from build123d import *

# Parameters (mm, degrees)
SKETCH_W     = 380
SKETCH_H     = 250
PAD_DEPTH    = 18
SKETCH001_W  = 284
SKETCH001_H  = 154
POCKET_DEPTH = 5
SKETCH004_R  = 1.55
HOLE_DEPTH   = 13.001


with BuildPart() as part:
    # Sketch → Pad (new body)
    with BuildSketch(Plane.XY):
        with Locations((190, 125)):
            Rectangle(SKETCH_W, SKETCH_H)
    extrude(amount=PAD_DEPTH)

    # Sketch001 (on Face6 of Pad) → Pocket (cut)
    with BuildSketch(Plane.XY.offset(18)):
        Polygon((30, 250), (30, 220), (0, 220), (0, 202), (30, 202), (30, 48), (0, 48), (0, 30), (30, 30), (30, 0), (48, 0), (48, 30), (332, 30), (332, 0), (350, 0), (350, 30), (380, 30), (380, 48), (350, 48), (350, 202), (380, 202), (380, 220), (350, 220), (350, 250), (332, 250), (332, 220), (48, 220), (48, 250), align=None)
        with Locations((190, 125)):
            Rectangle(SKETCH001_W, SKETCH001_H, mode=Mode.SUBTRACT)
    extrude(amount=-POCKET_DEPTH, mode=Mode.SUBTRACT)

    # Sketch004 (on Face6 of Pocket) → Hole (cut, through all)
    with BuildSketch(Plane.XY.offset(13)):
        with Locations((39, 39)):
            Circle(SKETCH004_R)
        with Locations((341, 39)):
            Circle(SKETCH004_R)
        with Locations((341, 211)):
            Circle(SKETCH004_R)
        with Locations((39, 211)):
            Circle(SKETCH004_R)
        with Locations((190, 211)):
            Circle(SKETCH004_R)
        with Locations((190, 39)):
            Circle(SKETCH004_R)
    extrude(amount=-HOLE_DEPTH, mode=Mode.SUBTRACT)


solid = part.part
Can you work these out from the model? Positions are in its coordinate system, mm. Give positions to 0.01 mm unless a question says otherwise; leave off trailing zeros. Order: outer loops, then holes, each group sorted by start corner. A loop starts at its lowest first (then second) coordinate and runs counter-clockwise, first axis right, second up. Notation, with made-up numbers: (-28, 74.5) - (-3, 74.5) arc R22 ccw to (-3, 89.5) - close; hole circle Ø8 at (81, 64). An arc over 180 degrees is marked (long way). Write each question's results on one line, items separated by ' | '.
1) I'm going to push a flat-ended pin straight in: pin 1 Ø4 at (x, z) = (361, 16) entering from -Y. Where does the tip first touch, or does it pass through?
Final values:
pin 1: stops at y = 0
2) Please list where these lines run through material, in increasing order: line 1 along X through (y, z) = (211, 9.5); line 2 along X through (y, z) = (12.5, 15); line 3 along Y through (x, z) = (190, 3.75). Write a range as [from, to].
Final values:
line 1: x = [0, 37.45], [40.55, 188.45], [191.55, 339.45], [342.55, 380] | line 2: x = [0, 30], [48, 332], [350, 380] | line 3: y = [0, 37.45], [40.55, 209.45], [212.55, 250]
3) Suppose I cut it at A-A, the plane y = 172.5. Write out the boundary of the cut face in (x, z).
Final values:
outline: (0, 0) - (380, 0) - (380, 18) - (350, 18) - (350, 13) - (332, 13) - (332, 18) - (48, 18) - (48, 13) - (30, 13) - (30, 18) - (0, 18) - close
4) If we mould it in two halves opening along X, with no side actions, what happens to faces 1 (the face through (0, 123, 9)), 2 (the face through (15, 15, 18)), 3 (the face through (380, 123, 9)), 4 (the face through (175, 42, 13))? For each: pulls with the +X half, pulls with the -X half, needs draft (parallel to the pull), parting line crosses it, or undercut.
Final values:
face 1: pulls with the -X half | face 2: needs draft | face 3: pulls with the +X half | face 4: undercut
5) Suppose I cut it at B-B, the plane x = 312.5. Write out the boundary of the cut face in (y, z), then the cut area to 3 significant figures.
Final values:
outline: (0, 0) - (250, 0) - (250, 18) - (220, 18) - (220, 13) - (202, 13) - (202, 18) - (48, 18) - (48, 13) - (30, 13) - (30, 18) - (0, 18) - close | area: 4,320 mm^2
